Source: three-view drawing plus pictorial views. Frame: mm from the lowest corner of the part. Coordinates: 2 decimals unless noted, no trailing zeros. Write each loop counter-clockwise with the first axis right and the second up, starting at its lowest first coordinate (ties: lowest second). Pieces come first, ordered by that corner, then holes. Notation, with made-up numbers: M 72.25,27.5 L 93.25,27.5 A30 ccw 93.25,61.5 Z; hole C 71,35 d9. An arc over 180 degrees is marked long. Use CSV: the item, a comma, the result in double quotes.
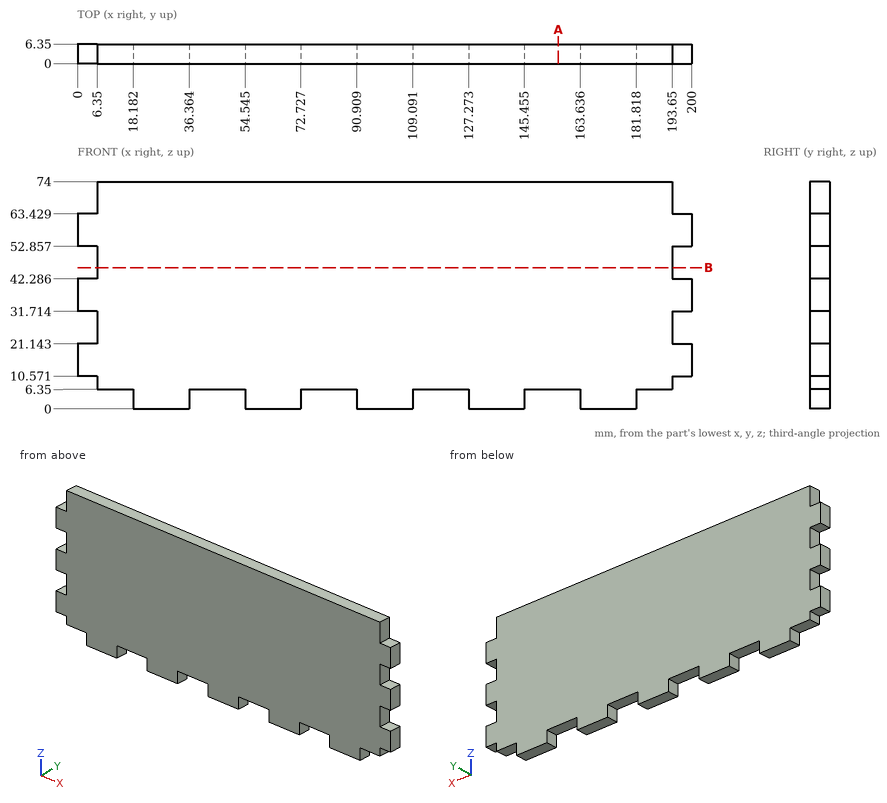
1. Material intervals for line 1 (X direction, y = 0.75, z = 30); line 2 (Z direction, x = 90, y = 1.5), sorted ascending. Write a range as [from, to].
Resolved:
line 1,"x = [6.35, 193.65]"
line 2,"z = [6.35, 74]"
2. Section A-A (x = 156.5). Return loops of the section in (y, z).
Resolved:
outline,"M 0,6.35 L 6.35,6.35 L 6.35,74 L 0,74 Z"
3. Section B-B (z = 46). Return loops of the section in (x, y), then the cut area to 3 significant figures.
Resolved:
outline,"M 6.35,0 L 193.65,0 L 193.65,6.35 L 6.35,6.35 Z"
area,"1,190 mm^2"
4. Contact query for flat-ended pins moving along their axis: pin 1 Ø1.9 at (y, z) = (2.5, 2.5) entering from -X; pin 2 Ø1.9 at (x, y) = (196.5, 2) entering from -Z; pin 3 Ø3 at (x, y) = (43.5, 4.5) entering from -Z. Output: stop coordinate, or through.
Resolved:
pin 1,"stops at x = 18.18"
pin 2,"stops at z = 10.57"
pin 3,"stops at z = 6.35"
